```python
from build123d import *

# Parameters (mm, degrees)
SKIZZE1_W                       = 195
SKIZZE1_H                       = 130
AUFSATZ_LINEAR_AUSTRAGEN1_DEPTH = 53
SKIZZE2_W                       = 139
SKIZZE2_H                       = 126
SCHNITT_LINEAR_AUSTRAGEN1_DEPTH = 50
SKIZZE3_W                       = 50
SKIZZE3_H                       = 42
SCHNITT_LINEAR_AUSTRAGEN2_DEPTH = 50
SKIZZE4_W                       = 50
SKIZZE4_H                       = 45
SCHNITT_LINEAR_AUSTRAGEN3_DEPTH = 50
SKIZZE5_W                       = 50
SKIZZE5_H                       = 35
SCHNITT_LINEAR_AUSTRAGEN4_DEPTH = 50
SKIZZE6_W                       = 195
SKIZZE6_H                       = 130
AUFSATZ_LINEAR_AUSTRAGEN2_DEPTH = 20
SKIZZE7_W                       = 35
SKIZZE7_H                       = 130
SCHNITT_LINEAR_AUSTRAGEN5_DEPTH = 20


with BuildPart() as part:
    # Skizze1 → Aufsatz-Linear austragen1 (new body)
    with BuildSketch(Plane(origin=(0, 0, -3), x_dir=(-1, 0, 0), z_dir=(0, 0, -1))):
        with Locations((-28.307004173, -3.528995936)):
            Rectangle(SKIZZE1_W, SKIZZE1_H)
    extrude(amount=-AUFSATZ_LINEAR_AUSTRAGEN1_DEPTH)

    # Skizze2 → Schnitt-Linear austragen1 (cut)
    with BuildSketch(Plane.XY.offset(50)):
        with Locations((2.307004173, -3.528995936)):
            Rectangle(SKIZZE2_W, SKIZZE2_H)
    extrude(amount=-SCHNITT_LINEAR_AUSTRAGEN1_DEPTH, mode=Mode.SUBTRACT)

    # Skizze3 → Schnitt-Linear austragen2 (cut)
    with BuildSketch(Plane.XY.offset(50)):
        with Locations((98.807004173, 38.471004064)):
            Rectangle(SKIZZE3_W, SKIZZE3_H)
    extrude(amount=-SCHNITT_LINEAR_AUSTRAGEN2_DEPTH, mode=Mode.SUBTRACT)

    # Skizze4 → Schnitt-Linear austragen3 (cut)
    with BuildSketch(Plane.XY.offset(50)):
        with Locations((98.807004173, -44.028995936)):
            Rectangle(SKIZZE4_W, SKIZZE4_H)
    extrude(amount=-SCHNITT_LINEAR_AUSTRAGEN3_DEPTH, mode=Mode.SUBTRACT)

    # Skizze5 → Schnitt-Linear austragen4 (cut)
    with BuildSketch(Plane.XY.offset(50)):
        with Locations((98.807004173, -2.028995936)):
            Rectangle(SKIZZE5_W, SKIZZE5_H)
    extrude(amount=-SCHNITT_LINEAR_AUSTRAGEN4_DEPTH, mode=Mode.SUBTRACT)

    # Skizze6 → Aufsatz-Linear austragen2 (add)
    with BuildSketch(Plane(origin=(0, 0, -3), x_dir=(-1, 0, 0), z_dir=(0, 0, -1))):
        with Locations((-28.307004173, -3.528995936)):
            Rectangle(SKIZZE6_W, SKIZZE6_H)
    extrude(amount=AUFSATZ_LINEAR_AUSTRAGEN2_DEPTH)

    # Skizze7 → Schnitt-Linear austragen5 (cut)
    with BuildSketch(Plane(origin=(0, 0, -23), x_dir=(-1, 0, 0), z_dir=(0, 0, -1))):
        with Locations((-85.807004173, -3.528995936)):
            Rectangle(SKIZZE7_W, SKIZZE7_H)
        with Locations((29.192995827, -3.528995936)):
            Rectangle(SKIZZE7_W, SKIZZE7_H)
    extrude(amount=-SCHNITT_LINEAR_AUSTRAGEN5_DEPTH, mode=Mode.SUBTRACT)


solid = part.part
```
For this review, take the finished solid that the model builds, in its own axes (mm). A direction names the side the tool comes from. Coordinates: 2 decimals unless noted, no trailing zeros. Write each loop counter-clockwise with the first axis right and the second up, starting at its lowest first coordinate (ties: lowest second). Pieces come first, ordered by that corner, then holes.
(1) Tool access review of faces 3 (the face through (98, 17.471, 25)), 4 (the face through (86, -3, -3)): name each direction out of +Z, -Z, +X, -X, +Y, -Y from which nothing blocks a thin tool from reaching the whole face with its end or side.
(2) Add section B-B on x = 76. Give the boundary of the cut face in (y, z), then the cut area to 3 significant figures.
(3) Add section D-D on y = -44. Give the boundary of the cut face in (x, z), then the cut area to 4 significant figures.
(4) For pin 1 Ø17.5 at (x, y) = (109, -3) entering from +Z, flat-tipped, find the tip position at first contact; note if it passes through.
(5) Wall thickness on probe 1 along X at (y, z) = (-37, 31.5); probe 2 along X at (y, z) = (-29, -16); probe 3 along Y at (x, z) = (93, 5): over which ranges is each line inside the solid? List them lowest first.
(6) Add section C-C on z = 43.5. Give the boundary of the cut face in (x, y), then the cut area to 3 significant figures.
(7) Add section A-A on z = -10.5. Give the boundary of the cut face in (x, y).
(8) The part is to be moulded in two halves that separate along X. For faces 1 (the face through (30, 61.471, 14)), 2 (the face through (-46.693, -4, -13)), say which applies: +X half, -X half, draft (parallel to the pull), parting line (faces both ways), or undercut.
Answer sheet:
1. face 3: +Z
1. face 4: -Z, +Y, -Y
2. outline: (-68.53, -3) - (61.47, -3) - (61.47, 50) - (59.47, 50) - (59.47, 0) - (17.47, 0) - (17.47, 50) - (15.47, 50) - (15.47, 0) - (-19.53, 0) - (-19.53, 50) - (-21.53, 50) - (-21.53, 0) - (-66.53, 0) - (-66.53, 50) - (-68.53, 50) - close
2. area: 790 mm2
3. outline: (-69.19, -23) - (-46.69, -23) - (-46.69, -3) - (-11.69, -3) - (-11.69, -23) - (68.31, -23) - (68.31, -3) - (103.31, -3) - (103.31, -23) - (125.81, -23) - (125.81, 50) - (123.81, 50) - (123.81, 0) - (73.81, 0) - (73.81, 50) - (71.81, 50) - (71.81, 0) - (-67.19, 0) - (-67.19, 50) - (-69.19, 50) - close
3. area: 3,385 mm2
4. pin 1: stops at z = 0
5. probe 1: x = -69.19 to -67.19, 71.81 to 73.81, 123.81 to 125.81
5. probe 2: x = -69.19 to -46.69, -11.69 to 68.31, 103.31 to 125.81
5. probe 3: y = -68.53 to -66.53, -21.53 to -19.53, 15.47 to 17.47, 59.47 to 61.47
6. outline: (-69.19, -68.53) - (125.81, -68.53) - (125.81, 61.47) - (-69.19, 61.47) - close; hole (-67.19, -66.53) - (71.81, -66.53) - (71.81, 59.47) - (-67.19, 59.47) - close; hole (73.81, -66.53) - (123.81, -66.53) - (123.81, -21.53) - (73.81, -21.53) - close; hole (73.81, -19.53) - (123.81, -19.53) - (123.81, 15.47) - (73.81, 15.47) - close; hole (73.81, 17.47) - (123.81, 17.47) - (123.81, 59.47) - (73.81, 59.47) - close
6. area: 1,740 mm2
7. outline: (-69.19, -68.53) - (-46.69, -68.53) - (-46.69, 61.47) - (-69.19, 61.47) - close; (-11.69, -68.53) - (68.31, -68.53) - (68.31, 61.47) - (-11.69, 61.47) - close; (103.31, -68.53) - (125.81, -68.53) - (125.81, 61.47) - (103.31, 61.47) - close
8. face 1: draft
8. face 2: undercut
